Build history of the part. All positions in model axes, mm. A direction names the side the tool comes from. Give positions to 0.01 mm unless a question says otherwise; leave off trailing zeros. Write each loop counter-clockwise with the first axis right and the second up, starting at its lowest first coordinate (ties: lowest second). Pieces come first, ordered by that corner, then holes. Notation, with made-up numbers: M 21,45.5 L 53,45.5 A19 cw 53,66.5 Z; hole C 39,85.25 d6. An arc over 180 degrees is marked long. Return JSON: item names as keys, results as strings. Group by question number.
Q1. Pull direction Z, two halves, no side cores. Call faces 5 (the flat face through (11.255, -3, 1)), 6 (the cylindrical face through (22.76, 79.33, 39.28)), 7 (the cylindrical face through (37.014, 79.331, 37.768)): +Z half, -Z half, draft (parallel to the pull), parting line (faces both ways), or undercut.
Q2. Wall check: probe 1 along Y at (x, z) = (11, 1); probe 2 along X at (y, z) = (-4, -38); probe 3 along X at (y, z) = (62, -34.5). Give the ranges that are in metal, low to high.
Q3. Band-saw the part on A-A, the plane z = 12.7. Give the cut face in (x, y), then the cut area to 3 significant figures.
Q4. Band-saw the part on B-B, the plane y = 29.5. Give the cut face in (x, z), then the cut area to 3 significant figures.
Q5. Tool access for faces 1 (the cylindrical face through (4.15, -3.22, -10.34)), 2 (the flat face through (-37, 76.2, -1)), 3 (the cylindrical face through (1.33, 79.33, -40.65)), 4 (the flat face through (20, 76.2, -1)): list every direction of +Z, -Z, +X, -X, +Y, -Y with a clear straight run to the whole face (end or side of a thin tool).
Q6. Band-saw the part on D-D, the plane x = -42. Give the cut face in (y, z).
Q7. Band-saw the part on C-C, the plane z = -38.1. Count the separate pieces of the cut face and the enclosed holes in it, then the cut area to 3 significant figures.
Q8. Flat gauge pins, fed straight in: pin 1 Ø12 at (y, z) = (23.5, 32) entering from -X; pin 2 Ø5 at (x, z) = (29, -15) entering from -Y; pin 3 Ø4.5 at (x, z) = (-36.65, -38.1) entering from -Y; pin 4 Ø12 at (y, z) = (19.5, 26.5) entering from +X. Where does each tip first touch, or does it go through?
Autodesk Inventor part; units mm, degrees
ref_plane "YZ Plane" through (0, 0, 0) normal (1, 0, 0) x (0, 1, 0)
ref_plane "XZ Plane" through (0, 0, 0) normal (0, 1, 0) x (-1, 0, 0)
ref_plane "XY Plane" through (0, 0, 0) normal (0, 0, 1) x (1, 0, 0)
sketch "Sketch1" plane through (0, 0, 0) normal (0, 1, 0) x (-1, 0, 0)
  line L0 (11.2547, 50.8) -> (-11.2547, 50.8)
  line L1 (-11.2547, 50.8) -> (-11.2547, -50.8)
  line L2 (-11.2547, -50.8) -> (11.2547, -50.8)
  line L3 (11.2547, -50.8) -> (11.2547, 50.8)
  line L4 (11.2547, 50.8) -> (-11.2547, -50.8) construction
  line L5 (-11.2547, 50.8) -> (11.2547, -50.8) construction
  point P0 (0, 0)
  dimension "d0" = 101.6
  dimension "d1" = 22.5095
extrude "Extrusion1" add sketch "Sketch1" against normal blind 6.35
sketch "Sketch2" plane through (0, 0, 0) normal (0, 1, 0) x (1, 0, 0)
  line L0 (11.2547, -50.8) -> (-11.2547, -50.8)
  line L1 (-11.2547, 50.8) -> (11.2547, 50.8)
  line L2 (-11.2547, -50.8) -> (-4.9047, -50.8)
  line L3 (-4.9047, -50.8) -> (-4.9047, 50.8)
  line L4 (-4.9047, 50.8) -> (-11.2547, 50.8)
  line L5 (-11.2547, 50.8) -> (-11.2547, -50.8)
  point P0 (0, 0)
  dimension "d4" = 6.35
extrude "Extrusion2" add sketch "Sketch2" along normal blind 76.2
sketch "Sketch3" plane through (0, 76.2, 0) normal (0, 1, 0) x (1, 0, 0)
  line L0 (11.2547, -50.8) -> (-11.2547, -50.8)
  line L1 (-11.2547, -50.8) -> (-62.0547, -50.8)
  line L2 (-62.0547, -50.8) -> (-62.0547, 50.8)
  line L3 (-62.0547, 50.8) -> (-11.2547, 50.8)
  line L4 (-11.2547, 50.8) -> (-11.2547, -50.8)
  line L5 (-4.9047, -50.8) -> (-4.9047, 50.8)
  line L6 (-4.9047, 50.8) -> (-11.2547, 50.8)
  line L7 (-11.2547, -50.8) -> (-4.9047, -50.8)
  line L8 (11.2547, -50.8) -> (11.2547, 50.8)
  line L9 (11.2547, 50.8) -> (-4.9047, 50.8)
  line L10 (-11.2547, -50.8) -> (-11.2547, 50.8)
  line L11 (-11.2547, -50.8) -> (-4.9047, -50.8)
  line L12 (-4.9047, -50.8) -> (-4.9047, 50.8)
  line L13 (-4.9047, 50.8) -> (-11.2547, 50.8)
  line L14 (-11.2547, 50.8) -> (-11.2547, -50.8)
  line L15 (-4.9047, -50.8) -> (45.8953, -50.8)
  line L16 (45.8953, -50.8) -> (45.8953, 50.8)
  line L17 (45.8953, 50.8) -> (-4.9047, 50.8)
  line L18 (-4.9047, 50.8) -> (-4.9047, -50.8)
  point P0 (0, 0)
  dimension "d7" = 50.8
  dimension "d8" = 50.8
extrude "Extrusion3" add sketch "Sketch3" along normal blind 6.35
sketch "Sketch4" plane through (0, 0, 0) normal (0, 1, 0) x (1, 0, 0)
  line L0 (-4.9047, -50.8) -> (11.2547, -50.8) construction
  line L1 (3.175, -50.8) -> (3.175, 50.8) construction
  line L2 (-11.2547, 50.8) -> (11.2547, 50.8) construction
  point P0 (0, 0)
  point P1 (3.175, -38.1)
  point P2 (3.175, -12.7)
  point P3 (3.175, 12.7)
  point P4 (3.175, 38.1)
  dimension "d11" = 12.7
  dimension "d14" = 25.4
hole "Hole1" at (3.175, 0, 38.1) at (3.175, 0, 12.7) at (3.175, 0, -12.7) at (3.175, 0, -38.1) direction (0, -1, 0) diameter 5.1054 end through all
sketch "Sketch5" plane through (0, 82.55, 0) normal (0, 1, 0) x (1, 0, 0)
  line L0 (-62.0547, 50.8) -> (-62.0547, -50.8) construction
  line L1 (-62.0547, -38.1) -> (42.9055, -38.1) construction
  line L2 (-55.7047, -38.1) -> (-55.7047, 38.1) construction
  point P0 (0, 0)
  point P1 (-36.6547, -38.1)
  point P2 (-36.6547, 38.1)
  point P3 (-17.6047, -38.1)
  point P4 (-17.6047, 38.1)
  point P5 (1.4453, -38.1)
  point P6 (1.4453, 38.1)
  point P7 (20.4953, -38.1)
  point P8 (20.4953, 38.1)
  point P9 (39.5453, -38.1)
  point P10 (39.5453, 38.1)
  point P11 (58.5953, -38.1)
  point P12 (58.5953, 38.1)
  dimension "d26" = 38.1
  dimension "d27" = 76.2
  dimension "d28" = 6.35
  dimension "d31" = 76.2
  dimension "d34" = 19.05
hole "Hole2" at (-55.7047, 82.55, 38.1) at (-55.7047, 82.55, -38.1) at (-36.6547, 82.55, 38.1) at (-36.6547, 82.55, -38.1) at (-17.6047, 82.55, 38.1) at (-17.6047, 82.55, -38.1) at (1.4453, 82.55, 38.1) at (1.4453, 82.55, -38.1) at (20.4953, 82.55, 38.1) at (20.4953, 82.55, -38.1) at (39.5453, 82.55, 38.1) at (39.5453, 82.55, -38.1) at (58.5953, 82.55, 38.1) at (58.5953, 82.55, -38.1) direction (0, -1, 0) diameter 5.1054 depth 6.35
equation "\"d0\" = BaseLength"
equation "\"d1\" = BaseWidth"
equation "\"d2\" = BaseThickness"
equation "\"d4\" = BackWidth"
equation "\"d5\" = BackHeight"
equation "\"d7\" = TopBackExtension"
equation "\"d8\" = TopFrontExtension"
equation "\"d9\" = TopThickness"
equation "\"d27\" = holeSpacingForMotorBracket"
equation "\"d28\" = offsetForBracketHoleFromEdge"
equation "\"BaseWidth\" = 22.50948"
equation "\"BaseLength\" = 101.6"
equation "\"BaseThickness\" = 6.35"
equation "\"BackWidth\" = 6.35"
equation "\"BackHeight\" = 76.2"
equation "\"TopBackExtension\" = 50.8"
equation "\"TopFrontExtension\" = 50.8"
equation "\"TopThickness\" = 6.35"
equation "\"offsetForFirstHole\" = 12.7"
equation "\"holeSpacingForMotorBracket\" = 76.2"
equation "\"offsetForBracketHoleFromEdge\" = 6.35"
equation "\"holeSpacingForVariationInMotorBracketHoles\" = 19.05"
properties part number "pullyBracket"
From the geometry:
{
 "1": {"face 5": "draft", "face 6": "undercut", "face 7": "undercut"},
 "2": {"probe 1": "y = -6.35 to 0, 76.2 to 82.55", "probe 2": "x = -11.25 to 0.62, 5.73 to 11.25", "probe 3": "x = -11.25 to -4.9"},
 "3": {"outline": "M -62.05,76.2 L -11.25,76.2 L -11.25,-6.35 L 0.62,-6.35 L 0.62,0 L -4.9,0 L -4.9,76.2 L 45.9,76.2 L 45.9,82.55 L -62.05,82.55 Z; M 5.73,-6.35 L 11.25,-6.35 L 11.25,0 L 5.73,0 Z", "area": "1,280 mm^2"},
 "4": {"outline": "M -11.25,-50.8 L -4.9,-50.8 L -4.9,50.8 L -11.25,50.8 Z", "area": "645 mm^2"},
 "5": {"face 1": "-Y", "face 2": "+Z, -Z, -X, -Y", "face 3": "+Y", "face 4": "+Z, -Z, +X"},
 "6": {"outline": "M 76.2,-50.8 L 82.55,-50.8 L 82.55,50.8 L 76.2,50.8 Z"},
 "7": {"separate pieces": "8", "enclosed holes": "0", "area": "1,090 mm^2"},
 "8": {"pin 1": "stops at x = -11.25", "pin 2": "stops at y = 76.2", "pin 3": "passes through", "pin 4": "stops at x = -4.9"}
}
